Geometry check sheet. Reference: the model listing, model coordinates, mm. Round coordinates to 2 decimals unless told otherwise and drop trailing zeros. Write each loop counter-clockwise with the first axis right and the second up, starting at its lowest first coordinate (ties: lowest second). Pieces come first, ordered by that corner, then holes. Notation, with made-up numbers: (-38.5, 48.25) -> (14.5, 48.25) arc R18 cw to (14.5, 58.25) -> close; hole circle Ø10 at (-1.75, -11). An arc over 180 degrees is marked (long way). Put each result on its own line as item: value. Start each with the question number.
from build123d import *

# Parameters (mm, degrees)
SKETCH1_W           = 5.4
SKETCH1_H           = 48.265
BOSS_EXTRUDE1_DEPTH = 5.4
SKETCH2_W           = 5.31872
SKETCH2_H           = 48.18372
BOSS_EXTRUDE2_DEPTH = 5.4


with BuildPart() as part:
    # Sketch1 → Boss-Extrude1 (new body)
    with BuildSketch(Plane.XY):
        Polygon((9.7125, -120.6625), (145.6875, -120.6625), (145.6875, -72.3975), (151.0875, -72.3975), (151.0875, -24.1325), (145.6875, -24.1325), (145.6875, 24.1325), (151.0875, 24.1325), (151.0875, 72.3975), (145.6875, 72.3975), (145.6875, 120.6625), (-145.6875, 120.6625), (-145.6875, 72.3975), (-151.0875, 72.3975), (-151.0875, 24.1325), (-145.6875, 24.1325), (-145.6875, -24.1325), (-151.0875, -24.1325), (-151.0875, -72.3975), (-145.6875, -72.3975), (-145.6875, -120.6625), (4.3125, -120.6625), (4.3125, 0), (9.7125, 0), align=None)
        with Locations((-128.5875, -48.265)):
            Rectangle(SKETCH1_W, SKETCH1_H, mode=Mode.SUBTRACT)
        with Locations((-128.5875, 48.265)):
            Rectangle(SKETCH1_W, SKETCH1_H, mode=Mode.SUBTRACT)
    extrude(amount=BOSS_EXTRUDE1_DEPTH)

    # Sketch2 → Boss-Extrude2 (add)
    with BuildSketch(Plane.XY.offset(5.4)):
        Polygon((-145.72814, -120.70314), (4.35314, -120.70314), (4.35314, -0.04064), (9.67186, -0.04064), (9.67186, -120.70314), (145.72814, -120.70314), (145.72814, -72.43814), (151.12814, -72.43814), (151.12814, -24.09186), (145.72814, -24.09186), (145.72814, 24.09186), (151.12814, 24.09186), (151.12814, 72.43814), (145.72814, 72.43814), (145.72814, 120.70314), (-145.72814, 120.70314), (-145.72814, 72.43814), (-151.12814, 72.43814), (-151.12814, 24.09186), (-145.72814, 24.09186), (-145.72814, -24.09186), (-151.12814, -24.09186), (-151.12814, -72.43814), (-145.72814, -72.43814), align=None)
        with Locations((-128.5875, 48.265)):
            Rectangle(SKETCH2_W, SKETCH2_H, mode=Mode.SUBTRACT)
        with Locations((-128.5875, -48.265)):
            Rectangle(SKETCH2_W, SKETCH2_H, mode=Mode.SUBTRACT)
    extrude(amount=-BOSS_EXTRUDE2_DEPTH)


solid = part.part
(1) Material ranges on L1, parallel to X at y = -46, z = 3.55; L2, parallel to X at y = 28.5, z = 1.6; L3, parallel to X at y = -4, z = 4.75, recorded low to high. Write a range as from..to.
(2) Sectioned sample at B-B (y = 50). Record the cut outline in (x, z), and give its area (3 significant figures).
(3) Sectioned sample at D-D (y = -13). Record the cut outline in (x, z), and give its area (3 significant figures).
(4) Go/stop test with flat-tipped pins: pin 1 Ø1.6 at (x, z) = (147, 4) entering from -Y; pin 2 Ø2.5 at (y, z) = (100.5, 3.5) entering from +X; pin 3 Ø2.5 at (x, z) = (148, 3) entering from +Y. Record where each tip stops, or that it passes through.
(5) Sectioned sample at C-C (z = 1.55). State how many separate pieces and enclosed holes the cut face has, and give its area (3 significant figures).
(6) Sectioned sample at A-A (y = -67). Record the cut outline in (x, z), and give its area (3 significant figures).
Found:
1. L1: -151.13..-131.25, -125.93..4.35, 9.67..151.13
1. L2: -151.13..-131.25, -125.93..151.13
1. L3: -145.73..4.35, 9.67..145.73
2. outline: (-151.13, 0) -> (-131.25, 0) -> (-131.25, 5.4) -> (-151.13, 5.4) -> close; (-125.93, 0) -> (151.13, 0) -> (151.13, 5.4) -> (-125.93, 5.4) -> close
2. area: 1,600 mm2
3. outline: (-145.73, 0) -> (4.35, 0) -> (4.35, 5.4) -> (-145.73, 5.4) -> close; (9.67, 0) -> (145.73, 0) -> (145.73, 5.4) -> (9.67, 5.4) -> close
3. area: 1,550 mm2
4. pin 1: y = -72.44
4. pin 2: x = 145.73
4. pin 3: y = 72.44
5. separate pieces: 1
5. enclosed holes: 2
5. area: 70,200 mm2
6. outline: (-151.13, 0) -> (-131.25, 0) -> (-131.25, 5.4) -> (-151.13, 5.4) -> close; (-125.93, 0) -> (4.35, 0) -> (4.35, 5.4) -> (-125.93, 5.4) -> close; (9.67, 0) -> (151.13, 0) -> (151.13, 5.4) -> (9.67, 5.4) -> close
6. area: 1,570 mm2
